Geometry: final body of the model. Coordinates: model frame, mm. Coordinates: 2 decimals unless noted, no trailing zeros. Order: outer loops, then holes, each group sorted by start corner. A loop starts at its lowest first (then second) coordinate and runs counter-clockwise, first axis right, second up. Notation, with made-up numbers: (-19, 20) -> (-8, 20) arc R17 cw to (-8, 51) -> close; hole circle Ø11 at (-21.75, 48). An arc over 180 degrees is marked (long way). Answer in a Markdown table with one row per item. Add a question column.
1) Section query B-B on z = 0. Return the cut outline in (x, y), then the cut area to 3 significant figures.
2) Section query A-A on x = 0. Return the cut outline in (y, z), then the cut area to 3 significant figures.
3) Section query C-C on y = -5.25. Return the cut outline in (x, z).
4) Section query D-D on y = -0.5. Return the cut outline in (x, z).
5) Ray query, line 1 (Z direction, x = 0, y = -2); line 2 (Z direction, x = 1.5, y = -3.5); line 3 (X direction, y = -2.25, z = 0.25). Return the intervals inside material, ascending. Write a range as from..to.
6) Contact query for flat-ended pins moving along their axis: P1, Ø4.5, axis at x = 0, z = 0, coming from the +Y side; P2, Ø2, axis at y = -2, z = 2, coming from the +X side; P3, Ø3, axis at y = -4.5, z = 3.5, coming from the +X side. Output: stop coordinate, or through.
```python
from build123d import *

# Parameters (mm, degrees)
F0_R     = 6
F0_R_2   = 1.75
F1_DEPTH = 6.8
F2_R     = 1
F3_R     = 1


with BuildPart() as f1:
    # F0 (on Front) → F1 (new body)
    with BuildSketch(Plane.XZ):
        Circle(F0_R)
        Circle(F0_R_2, mode=Mode.SUBTRACT)
    extrude(amount=F1_DEPTH)

    # F2
    f2_edges = [f1.edges().sort_by_distance(p)[0] for p in [
        (-6, -6.8, 0),
        (-6, 0, 0),
    ]]
    fillet(f2_edges, radius=F2_R)

    # F3
    f3_edges = [f1.edges().sort_by_distance(p)[0] for p in [
        (-1.75, -6.8, 0),
        (-1.75, 0, 0),
    ]]
    fillet(f3_edges, radius=F3_R)


solid = f1.part
```
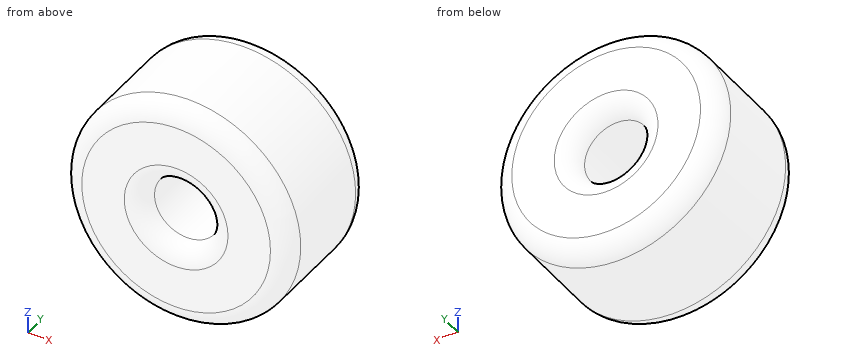
Result:
| question | item | result |
|---|---|---|
| 1 | outline | (-6, -5.8) arc R1 ccw to (-5, -6.8) -> (-2.75, -6.8) arc R1 ccw to (-1.75, -5.8) -> (-1.75, -1) arc R1 ccw to (-2.75, 0) -> (-5, 0) arc R1 ccw to (-6, -1) -> close; (1.75, -5.8) arc R1 ccw to (2.75, -6.8) -> (5, -6.8) arc R1 ccw to (6, -5.8) -> (6, -1) arc R1 ccw to (5, 0) -> (2.75, 0) arc R1 ccw to (1.75, -1) -> close |
| 1 | area | 56.1 mm2 |
| 2 | outline | (-6.8, -5) arc R1 ccw to (-5.8, -6) -> (-1, -6) arc R1 ccw to (0, -5) -> (0, -2.75) arc R1 ccw to (-1, -1.75) -> (-5.8, -1.75) arc R1 ccw to (-6.8, -2.75) -> close; (-6.8, 2.75) arc R1 ccw to (-5.8, 1.75) -> (-1, 1.75) arc R1 ccw to (0, 2.75) -> (0, 5) arc R1 ccw to (-1, 6) -> (-5.8, 6) arc R1 ccw to (-6.8, 5) -> close |
| 2 | area | 56.1 mm2 |
| 3 | outline | circle Ø12 at (0, 0); hole circle Ø3.5 at (0, 0) |
| 4 | outline | circle Ø11.73 at (0, 0); hole circle Ø3.77 at (0, 0) |
| 5 | line 1 | -6..-1.75, 1.75..6 |
| 5 | line 2 | -5.81..-0.9, 0.9..5.81 |
| 5 | line 3 | -5.99..-1.73, 1.73..5.99 |
| 6 | P1 | y = -0.13 |
| 6 | P2 | x = 5.92 |
| 6 | P3 | x = 5.66 |
